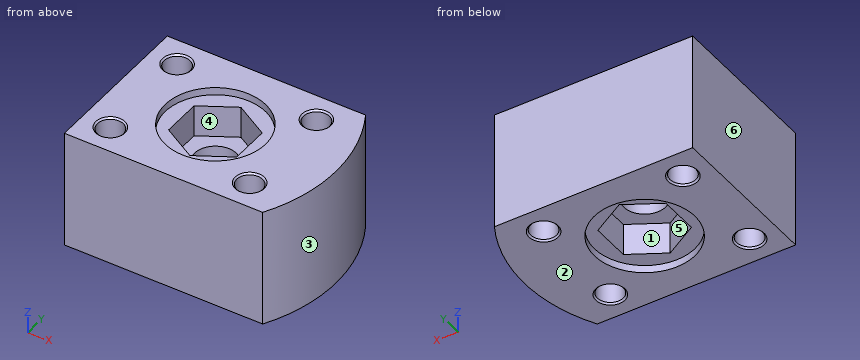
Autodesk Fusion 360 part; units mm, degrees
sketch "Sketch1" plane through (0, 0, 0) normal (0, 0, 1) x (1, 0, 0)
  circle A0 centre (0, 0) radius 12.6
  line L0 (-25, 19.9) -> (-25, -19.9)
  line L1 (-25, 19.9) -> (24.8138, 19.9)
  line L2 (-25, -19.9) -> (24.8138, -19.9)
  circle A1 centre (0, 0) radius 5.25
  arc A2 (24.8138, -19.9) -> (24.8138, 19.9) centre (-10, 0) ccw
  line L3 (0, 0) -> (-10, 0) construction
  line L4 (8.55, 4.9363) -> (0, 9.8727)
  line L5 (0, 9.8727) -> (-8.55, 4.9363)
  line L6 (-8.55, 4.9363) -> (-8.55, -4.9363)
  line L7 (-8.55, -4.9363) -> (0, -9.8727)
  line L8 (0, -9.8727) -> (8.55, -4.9363)
  line L9 (8.55, -4.9363) -> (8.55, 4.9363)
  circle A3 centre (-18, 12.9) radius 3.25
  circle A4 centre (-18, -12.9) radius 3.25
  circle A5 centre (17, -12.9) radius 3.25
  circle A6 centre (17, 12.9) radius 3.25
  line L10 (-18, 12.9) -> (17, 12.9) construction
  line L11 (17, 12.9) -> (17, -12.9) construction
  line L12 (17, -12.9) -> (-18, -12.9) construction
  dimension "d1" = 25.2
  dimension "d3" = 19.9
  dimension "d4" = 19.9
  dimension "d7" = 10.5
  dimension "d8" = 40.1
  dimension "d10" = 17.1
  dimension "d19" = 7
  dimension "d20" = 6.5
  dimension "d22" = 7
  dimension "d23" = 35
  dimension "d28" = 18
  dimension "d29" = 10
  dimension "d30" = 25
extrude "Extrude1" add sketch "Sketch1" along normal mid plane 29.8 contours L0 L1 L2 A2 makes body 1
extrude "Extrude3" add sketch "Sketch1" along normal mid plane 26 contours A0 bodies 1
extrude "Extrude4" add sketch "Sketch1" along normal mid plane 10 contours L4 L5 L6 L7 L8 L9 bodies 1
extrude "Extrude5" add sketch "Sketch1" along normal blind 5 and the other way blind 0 contours A3 | A4 | A5 | A6 bodies 1
copy_body "Body->Comp1" bodies 1 removing the originals makes body 2 in component "side brace lwr mount nut insert"
chamfer "Chamfer1" distance 0.4 angle 45 8 edges at (13.9699, 14.0753, 14.9) (-21.0301, 14.0753, 14.9) (-21.0301, -11.7247, 14.9) (13.9699, -11.7247, 14.9) (13.9699, -14.0753, -14.9) (-21.0301, 11.7247, -14.9) (13.9699, 11.7247, -14.9) (-21.0301, -14.0753, -14.9) on bodies 2 in component "side brace lwr mount nut insert"
component "side brace lwr mount nut insert" placed x (1, 0, 0) y (0, 1, 0) z (0, 0, 1) at (0, 0, 0)
equation "d4 = d3"
Part model, mm, in its own coordinate system. Face numbers are marked on the shaded views. A direction names the side the tool comes from. Give positions to 0.01 mm unless a question says otherwise; leave off trailing zeros. Write each loop counter-clockwise with the first axis right and the second up, starting at its lowest first coordinate (ties: lowest second). Pieces come first, ordered by that corner, then holes.
1) Cut at D-D on z = 3. Write the cut outline in (x, y), then the cut area to 3 significant figures.
Resolved:
outline: (-25, -19.9) - (24.81, -19.9) arc R40.1 ccw to (24.81, 19.9) - (-25, 19.9) - close; hole circle Ø10.5 at (0, 0)
area: 2,040 mm2
2) Cut at C-C on x = 17. Write the cut outline in (y, z).
Resolved:
outline: (-19.9, -14.9) - (-16.55, -14.9) - (-16.15, -14.5) - (-16.15, 0) - (-9.65, 0) - (-9.65, -14.5) - (-9.25, -14.9) - (9.25, -14.9) - (9.65, -14.5) - (9.65, 0) - (16.15, 0) - (16.15, -14.5) - (16.55, -14.9) - (19.9, -14.9) - (19.9, 14.9) - (16.55, 14.9) - (16.15, 14.5) - (16.15, 5) - (9.65, 5) - (9.65, 14.5) - (9.25, 14.9) - (-9.25, 14.9) - (-9.65, 14.5) - (-9.65, 5) - (-16.15, 5) - (-16.15, 14.5) - (-16.55, 14.9) - (-19.9, 14.9) - close
3) Which spindle directions (+Z, -Z, +X, -X, +Y, -Y) get a long thin tool onto all of the face, cutting with end or side? Do the marked faces 4, 5 and 6. Say none if no direction does.
Resolved:
face 4: +Z
face 5: -Z
face 6: +Z, -Z, -X, +Y, -Y
4) Cut at A-A on y = 0. Write the cut outline in (x, z), then the cut area to 3 significant figures.
Resolved:
outline: (-25, -14.9) - (-12.6, -14.9) - (-12.6, -13) - (-8.55, -13) - (-8.55, -5) - (-5.25, -5) - (-5.25, 5) - (-8.55, 5) - (-8.55, 13) - (-12.6, 13) - (-12.6, 14.9) - (-25, 14.9) - close; (5.25, -5) - (8.55, -5) - (8.55, -13) - (12.6, -13) - (12.6, -14.9) - (30.1, -14.9) - (30.1, 14.9) - (12.6, 14.9) - (12.6, 13) - (8.55, 13) - (8.55, 5) - (5.25, 5) - close
area: 1,170 mm2
5) Two-plate mould, pull along X, no slides. Class the marked faces 1, 2 and 3: released by +X, released by -X, zero draft, split by the parting line, or undercut.
Resolved:
face 1: undercut
face 2: zero draft
face 3: released by +X
6) Cut at B-B on z = 9. Write the cut outline in (x, y), then the cut area to 3 significant figures.
Resolved:
outline: (-25, -19.9) - (24.81, -19.9) arc R40.1 ccw to (24.81, 19.9) - (-25, 19.9) - close; hole circle Ø6.5 at (-18, -12.9); hole circle Ø6.5 at (-18, 12.9); hole (-8.55, -4.94) - (0, -9.87) - (8.55, -4.94) - (8.55, 4.94) - (0, 9.87) - (-8.55, 4.94) - close; hole circle Ø6.5 at (17, -12.9); hole circle Ø6.5 at (17, 12.9)
area: 1,740 mm2
7) Probe L1, parallel to Y at x = -18, z = -4.25; L2, parallel to Z at x = 10.5, y = -3; L3, parallel to Y at x = -0.5, z = 3.25. List the from-to ranges inside material, lowest first.
Resolved:
L1: y = -19.9 to -16.15, -9.65 to 9.65, 16.15 to 19.9
L2: z = -13 to 13
L3: y = -19.9 to -5.23, 5.23 to 19.9
8) Pin check, flat tips, straight feed: pin 1 (12.5 mm diameter, centred on x = 1.5, y = 0.5, fed in from -Z); pin 2 (1.9 mm diameter, centred on x = -18, y = 14.5, fed in from -Z); pin 3 (3 mm diameter, centred on x = 17, y = -12, fed in from +Z). Stop position of each tip, or through.
Resolved:
pin 1: stops at z = -5
pin 2: stops at z = 0
pin 3: stops at z = 5
